Autodesk Inventor part; units mm, degrees
ref_plane "YZ Plane" through (0, 0, 0) normal (1, 0, 0) x (0, 1, 0)
ref_plane "XZ Plane" through (0, 0, 0) normal (0, 1, 0) x (-1, 0, 0)
ref_plane "XY Plane" through (0, 0, 0) normal (0, 0, 1) x (1, 0, 0)
sketch "スケッチ1" plane through (0, 0, 0) normal (0, 0, 1) x (1, 0, 0)
  line L0 (-10, 10) -> (10, 10)
  line L1 (10, 10) -> (10, -10)
  line L2 (10, -10) -> (-10, -10)
  line L3 (-10, -10) -> (-10, 10)
  point P0 (0, 0)
  dimension "d0" = 20
  dimension "d1" = 10
  dimension "d2" = 20
  dimension "d3" = 10
extrude "押し出し1" add sketch "スケッチ1" along normal blind 21.8
sketch "スケッチ2" plane through (0, 0, 21.8) normal (0, 0, 1) x (1, 0, 0)
  point P0 (0, 0)
  point P1 (-7.2, 7.5)
  point P2 (-7.2, -7.5)
  point P3 (7.2, -7.5)
  point P4 (7.2, 7.5)
  dimension "d6" = 14.4
  dimension "d7" = 14.4
  dimension "d8" = 15
  dimension "d9" = 15
  dimension "d10" = 7.2
  dimension "d11" = 7.2
  dimension "d12" = 7.5
  dimension "d13" = 7.5
hole "Hole1" at (-7.2, 7.5, 21.8) at (-7.2, -7.5, 21.8) at (7.2, -7.5, 21.8) at (7.2, 7.5, 21.8) direction (0, 0, -1) diameter 2.013 end through all
sketch "スケッチ3" plane through (-10, -10, 0) normal (0, -1, 0) x (1, 0, 0)
  line L0 (20, 21.8) -> (0, 21.8)
  line L1 (20, 0) -> (20, 21.8)
  circle A0 centre (10, 10.9) radius 1.5
  line L2 (9.75, 15.9) -> (10.25, 15.9)
  line L3 (10.25, 15.9) -> (10.25, 5.9)
  line L4 (10.25, 5.9) -> (9.75, 5.9)
  line L5 (9.75, 5.9) -> (9.75, 15.9)
  point P0 (10, 0)
  dimension "d21" = 3
  dimension "d22" = 10.9
  dimension "d23" = 10
  dimension "d24" = 10
  dimension "d25" = 0.5
  dimension "d26" = 0.25
  dimension "d27" = 5
extrude "押し出し2" cut sketch "スケッチ3" against normal blind 15
equation "\"d26\" = 0.5 * d25"
equation "\"d27\" = 0.5 * d24"
properties part number "JointD1"
The model under review builds one solid part; all positions refer to its coordinate system, in mm. A direction names the side the tool comes from. Give positions to 0.01 mm unless a question says otherwise; leave off trailing zeros. Write each loop counter-clockwise with the first axis right and the second up, starting at its lowest first coordinate (ties: lowest second). Pieces come first, ordered by that corner, then holes. Notation, with made-up numbers: (59, 9) - (66, 9) arc R26 cw to (66, 26) - close; hole circle Ø11 at (22.5, -23). An arc over 180 degrees is marked (long way). Answer in a Markdown table with one row per item. Add a question column.
1. Draft analysis for pull direction Y (two halves, no side actions). For faces 1 (the cylindrical face through (7.59, -8.43, 10.75)), 2 (the flat face through (2, -10, 11)), 3 (the flat face through (10, 0, 11)), state which applies: +Y half, -Y half, draft (parallel to the pull), parting line (faces both ways), or undercut.
2. We need section C-C on z = 4.75. Write out the cut boundary in (x, y), then the cut area to 3 significant figures.
3. We need section D-D on x = -7.2. Write out the cut boundary in (y, z).
4. We need section B-B on y = 7.5. Write out the cut boundary in (x, z), then the cut area to 3 significant figures.
5. Tool access review of faces 4 (the flat face through (-0.25, -3, 14)), 5 (the flat face through (-10, 0, 11)): name each direction out of +Z, -Z, +X, -X, +Y, -Y from which nothing blocks a thin tool from reaching the whole face with its end or side.
6. Wall thickness on line 1 along X through (y, z) = (7.5, 16); line 2 along X through (y, z) = (-7.5, 6.5); line 3 along X through (y, z) = (-7.5, 11): over which ranges is each line inside the solid? List them lowest first. Write a range as [from, to].
7. Insertion check: P1, Ø2.5, axis at x = -7.2, y = -7.5, coming from the +Z side. The pin has a flat end and moves straight along its axis. Give the tip position at first contact, or say it passes through.
8. We need section A-A on y = -7.5. Write out the cut boundary in (x, z), then the cut area to 3 significant figures.
Ans:
| question | item | result |
|---|---|---|
| 1 | face 1 | undercut |
| 1 | face 2 | -Y half |
| 1 | face 3 | draft |
| 2 | outline | (-10, -10) - (10, -10) - (10, 10) - (-10, 10) - close; hole circle Ø2.01 at (-7.2, -7.5); hole circle Ø2.01 at (-7.2, 7.5); hole circle Ø2.01 at (7.2, -7.5); hole circle Ø2.01 at (7.2, 7.5) |
| 2 | area | 387 mm^2 |
| 3 | outline | (-10, 0) - (-8.51, 0) - (-8.51, 21.8) - (-10, 21.8) - close; (-6.49, 0) - (6.49, 0) - (6.49, 21.8) - (-6.49, 21.8) - close; (8.51, 0) - (10, 0) - (10, 21.8) - (8.51, 21.8) - close |
| 4 | outline | (-10, 0) - (-8.21, 0) - (-8.21, 21.8) - (-10, 21.8) - close; (-6.19, 0) - (6.19, 0) - (6.19, 21.8) - (-6.19, 21.8) - close; (8.21, 0) - (10, 0) - (10, 21.8) - (8.21, 21.8) - close |
| 4 | area | 348 mm^2 |
| 5 | face 4 | -Y |
| 5 | face 5 | +Z, -Z, -X, +Y, -Y |
| 6 | line 1 | x = [-10, -8.21], [-6.19, 6.19], [8.21, 10] |
| 6 | line 2 | x = [-10, -8.21], [-6.19, -0.25], [0.25, 6.19], [8.21, 10] |
| 6 | line 3 | x = [-10, -8.21], [-6.19, -1.5], [1.5, 6.19], [8.21, 10] |
| 7 | P1 | stops at z = 21.8 |
| 8 | outline | (-10, 0) - (-8.21, 0) - (-8.21, 21.8) - (-10, 21.8) - close; (-6.19, 0) - (6.19, 0) - (6.19, 21.8) - (-6.19, 21.8) - close; (8.21, 0) - (10, 0) - (10, 21.8) - (8.21, 21.8) - close; hole (-0.25, 5.9) - (0.25, 5.9) - (0.25, 9.42) arc R1.5 ccw to (0.25, 12.38) - (0.25, 15.9) - (-0.25, 15.9) - (-0.25, 12.38) arc R1.5 ccw to (-0.25, 9.42) - close |
| 8 | area | 338 mm^2 |
